Can you work these out from the model? Positions are in its coordinate system, mm. Round coordinates to 2 decimals unless told otherwise and drop trailing zeros.
(1) Thinking about a two-plate mould opening in Z: for faces 1 (the face through (-91.981, 902.847, -44.084)), 2 (the face through (-90.502, 948, -44)), which applies, released by +Z, released by -Z, zero draft, split by the parting line, or undercut?
(2) Will this pin go through, and if not, where does the flat tip stop? pin 1 Ø4 at (y, z) = (1105.63, -72) entering from +X.
(3) If I drill on line 1 along Y through (x, z) = (-92.5, -43.5); line 2 along Y through (x, z) = (-91.5, -36); line 3 along Y through (x, z) = (-92.4, -12.5), over which ranges is the centre line in solid material (lowest first)?
(4) I want a section at A-A on x = -92.3. Give the number of separate pieces and of enclosed holes in the cut face, plus the area to 3 significant figures.
from build123d import *

# Parameters (mm, degrees)
CROQUIS3_W              = 90
CROQUIS3_H              = 482
CROQUIS3_R              = 2.5
CROQUIS3_R_2            = 6
CROQUIS3_R_3            = 1.5
CROQUIS3_R_4            = 5
CROQUIS3_R_5            = 2
SALIENTE_EXTRUIR1_DEPTH = 3


with BuildPart() as part:
    # Croquis3 → Saliente-Extruir1 (new body)
    with BuildSketch(Plane.ZY.offset(90.501614904)):
        with Locations((-43, 944.628389678)):
            Rectangle(CROQUIS3_W, CROQUIS3_H)
        with Locations((-72, 1105.628389678)):
            Circle(CROQUIS3_R, mode=Mode.SUBTRACT)
        with Locations((-14, 1105.628389678)):
            Circle(CROQUIS3_R, mode=Mode.SUBTRACT)
        with Locations((-72, 1013.628389678)):
            Circle(CROQUIS3_R, mode=Mode.SUBTRACT)
        with Locations((-14, 1013.628389678)):
            Circle(CROQUIS3_R, mode=Mode.SUBTRACT)
        with Locations((-36, 944.628389678)):
            Circle(CROQUIS3_R_2, mode=Mode.SUBTRACT)
        with Locations((-29.136829367, 936.116673787)):
            Circle(CROQUIS3_R_3, mode=Mode.SUBTRACT)
        with Locations((-43, 928.11276849)):
            Circle(CROQUIS3_R_3, mode=Mode.SUBTRACT)
        with Locations((-29.136829367, 952.124484381)):
            Circle(CROQUIS3_R_3, mode=Mode.SUBTRACT)
        with Locations((-43, 960.128389678)):
            Circle(CROQUIS3_R_3, mode=Mode.SUBTRACT)
        with Locations((-56.863170633, 952.124484381)):
            Circle(CROQUIS3_R_3, mode=Mode.SUBTRACT)
        with Locations((-56.863170633, 936.116673787)):
            Circle(CROQUIS3_R_3, mode=Mode.SUBTRACT)
        with Locations((-43, 907.728389678)):
            Circle(CROQUIS3_R_4, mode=Mode.SUBTRACT)
        with Locations((-14, 875.628389678)):
            Circle(CROQUIS3_R, mode=Mode.SUBTRACT)
        with Locations((-27.458426503, 860.118311041)):
            Circle(CROQUIS3_R_5, mode=Mode.SUBTRACT)
        with Locations((-27.458426503, 892.118311041)):
            Circle(CROQUIS3_R_5, mode=Mode.SUBTRACT)
        with Locations((-14, 783.628389678)):
            Circle(CROQUIS3_R, mode=Mode.SUBTRACT)
        with Locations((-27.458426503, 768.118311041)):
            Circle(CROQUIS3_R_5, mode=Mode.SUBTRACT)
        with Locations((-27.458426503, 800.118311041)):
            Circle(CROQUIS3_R_5, mode=Mode.SUBTRACT)
        with Locations((-59.458426503, 768.118311041)):
            Circle(CROQUIS3_R_5, mode=Mode.SUBTRACT)
        with Locations((-72, 783.628389678)):
            Circle(CROQUIS3_R, mode=Mode.SUBTRACT)
        with Locations((-59.458426503, 800.118311041)):
            Circle(CROQUIS3_R_5, mode=Mode.SUBTRACT)
        with Locations((-59.458426503, 860.118311041)):
            Circle(CROQUIS3_R_5, mode=Mode.SUBTRACT)
        with Locations((-72, 875.628389678)):
            Circle(CROQUIS3_R, mode=Mode.SUBTRACT)
        with Locations((-59.458426503, 892.118311041)):
            Circle(CROQUIS3_R_5, mode=Mode.SUBTRACT)
        with BuildLine():
            Line((-59.458426503, 887.421766265), (-59.458426503, 864.814855817))
            ThreePointArc((-59.458426503, 864.814855817), (-63.048426503, 876.118311041), (-59.458426503, 887.421766265))
        make_face(mode=Mode.SUBTRACT)
        Polygon((-55.641915092, 891.4588034), (-55.458426503, 860.633864006), (-51.458426503, 858.236250198), (-51.458426503, 894.000371885), align=None, mode=Mode.SUBTRACT)
        Polygon((-47.458426503, 895.29559187), (-47.458426503, 856.941030212), (-43.458426503, 856.528311041), (-43.458426503, 895.708311041), align=None, mode=Mode.SUBTRACT)
        Polygon((-39.458426503, 856.941030212), (-35.458426503, 858.236250198), (-35.458426503, 894.000371885), (-39.458426503, 895.29559187), align=None, mode=Mode.SUBTRACT)
        Polygon((-31.458426503, 860.633864006), (-31.274937914, 891.4588034), (-27.458426503, 887.421766265), (-27.458426503, 864.814855817), align=None, mode=Mode.SUBTRACT)
        Polygon((-27.458426503, 772.814855817), (-31.274937914, 768.777818683), (-31.458426503, 799.602758077), (-27.458426503, 795.421766265), align=None, mode=Mode.SUBTRACT)
        Polygon((-35.458426503, 766.236250198), (-39.458426503, 764.941030212), (-39.458426503, 803.29559187), (-35.458426503, 802.000371885), align=None, mode=Mode.SUBTRACT)
        Polygon((-43.458426503, 764.528311041), (-47.458426503, 764.941030212), (-47.458426503, 803.29559187), (-43.458426503, 803.708311041), align=None, mode=Mode.SUBTRACT)
        Polygon((-51.458426503, 766.236250198), (-55.641915092, 768.777818683), (-55.458426503, 799.602758077), (-51.458426503, 802.000371885), align=None, mode=Mode.SUBTRACT)
        with BuildLine():
            Line((-59.458426503, 795.421766265), (-59.458426503, 772.814855817))
            ThreePointArc((-59.458426503, 772.814855817), (-63.048426503, 784.118311041), (-59.458426503, 795.421766265))
        make_face(mode=Mode.SUBTRACT)
    extrude(amount=SALIENTE_EXTRUIR1_DEPTH)


solid = part.part
Filled sheet:
1. face 1: undercut
1. face 2: zero draft
2. pin 1: passes through
3. line 1: y = 703.63 to 764.53, 803.7 to 856.53, 895.7 to 902.75, 912.7 to 926.7, 929.53 to 958.71, 961.54 to 1185.63
3. line 2: y = 703.63 to 766.06, 802.18 to 858.06, 894.18 to 938.63, 950.63 to 1185.63
3. line 3: y = 703.63 to 781.63, 785.63 to 873.63, 877.63 to 1011.63, 1015.63 to 1103.63, 1107.63 to 1185.63
4. separate pieces: 1
4. enclosed holes: 34
4. area: 41,700 mm2
